Autodesk Inventor part; units mm, degrees
ref_plane "YZ Plane" through (0, 0, 0) normal (1, 0, 0) x (0, 1, 0)
ref_plane "XZ Plane" through (0, 0, 0) normal (0, 1, 0) x (-1, 0, 0)
ref_plane "XY Plane" through (0, 0, 0) normal (0, 0, 1) x (1, 0, 0)
sketch "Skizze2" plane through (0, 0, 0) normal (0, 1, 0) x (-1, 0, 0)
  line L0 (18.5, 0) -> (9.25, -16.0215)
  line L1 (9.25, -16.0215) -> (-9.25, -16.0215)
  line L2 (-9.25, -16.0215) -> (-18.5, 0)
  line L3 (-18.5, 0) -> (-9.25, 16.0215)
  line L4 (-9.25, 16.0215) -> (9.25, 16.0215)
  line L5 (9.25, 16.0215) -> (18.5, 0)
  point P0 (0, 0)
  point P1 (0, 0)
  dimension "d8" = 37
extrude "Extrusion1" add sketch "Skizze2" along normal blind 5
sketch "Skizze4" plane through (0, 0, 0) normal (0, 0, 1) x (1, 0, 0)
  line L0 (9.25, 5) -> (-9.25, 5)
  line L1 (-9.25, 5) -> (-18.5, 5)
  line L2 (18.5, 5) -> (9.25, 5)
  arc A0 (-18.5, 5) -> (-13.5631, 9.2083) centre (-18.5, 10) ccw
  line L3 (-13.5631, 9.2083) -> (-11.8486, 19.9)
  arc A1 (0, 30) -> (-11.8486, 19.9) centre (0, 18) ccw
  line L4 (0, 30) -> (0, 0)
  line L5 (9.25, 0) -> (-9.25, 0)
  point P0 (0, 5)
  dimension "d11" = 12
  dimension "d12" = 5
  dimension "d13" = 30
revolve "Umdrehung1" add sketch "Skizze4" angle 360 about axis through (0, 30, 0) along (0, -1, 0)
sketch "Skizze5" plane through (0, 0, 0) normal (0, -1, 0) x (1, 0, 0)
  line L0 (-9.25, 16.0215) -> (9.25, 16.0215)
  line L1 (-18.5, 0) -> (-9.25, 16.0215)
  line L2 (-9.25, -16.0215) -> (-18.5, 0)
  line L3 (9.25, -16.0215) -> (-9.25, -16.0215)
  line L4 (18.5, 0) -> (9.25, -16.0215)
  line L5 (9.25, 16.0215) -> (18.5, 0)
  arc A0 (-18.5, 0) -> (-9.25, -16.0215) centre (0, 0) ccw
  arc A1 (-9.25, 16.0215) -> (-18.5, 0) centre (0, 0) ccw
  arc A2 (9.25, 16.0215) -> (-9.25, 16.0215) centre (0, 0) ccw
  arc A3 (18.5, 0) -> (9.25, 16.0215) centre (0, 0) ccw
  arc A4 (9.25, -16.0215) -> (18.5, 0) centre (0, 0) ccw
  line L6 (9.25, -16.0215) -> (-9.25, -16.0215)
  arc A5 (-9.25, -16.0215) -> (9.25, -16.0215) centre (0, 0) ccw
  point P0 (0, 0)
extrude "Extrusion4" cut sketch "Skizze5" against normal up to surface contours A2 L0 | L1 A1 | A3 L5 | L2 A0 | A4 L4 | L3 A5
sketch "Skizze6" plane through (0, 0, 0) normal (0, -1, 0) x (1, 0, 0)
  point P0 (0, 0)
  point P1 (0, 0)
hole "Bohrung1" at (0, 0, 0) direction (0, 1, 0) diameter 8.376 depth 25 tip angle 118
properties part number "Spinner" material "Bronze, Cast"
Work out the finished part from the listing and answer in its coordinate system (mm). A direction names the side the tool comes from. Round coordinates to 2 decimals unless told otherwise and drop trailing zeros. Write each loop counter-clockwise with the first axis right and the second up, starting at its lowest first coordinate (ties: lowest second). Pieces come first, ordered by that corner, then holes.
1) A tool of negligible diameter and unlimited length cuts with its end or side. For faces 4 (the cylindrical face through (-2.83, 12.675, 3.087)), 5 (the flat face through (13.94, 2.79, 7.9)), from which of +Z, -Z, +X, -X, +Y, -Y can it reach the whole face along a straight path? Write none if from no direction.
2) A cutting plane is placed at A-A (y = 3). Give the vertices of the cut face in (x, z).
3) Straight lines are drawn through the part: line 1 (Z direction, x = 1, y = 23.5); line 2 (Z direction, x = 0, y = 8.75); line 3 (X direction, y = 15.5, z = 0). For each, find the intervals that lie inside material, in ascending order.
4) Given pin 1 Ø1 at (y, z) = (16, 4) entering from +X; pin 2 Ø3 at (x, y) = (-6.5, 25) entering from -Z; pin 3 Ø6 at (x, z) = (-12, -7) entering from +Y; pin 4 Ø3 at (x, y) = (14, 20) entering from -Z, each flat-ended and moving along its own axis, determine where each tip first touches the part or whether it passes through.
5) The mould has two halves that part along Z. Classify faces 1 (the conical face through (0.49, 27.08, 0.54)), 2 (the flat face through (0, 3, 16.022)), 3 (the flat face through (-13.94, 2.79, -7.9)): pulls with the +Z half, pulls with the -Z half, needs draft (parallel to the pull), parting line crosses it, or undercut.
6) A cutting plane is placed at B-B (y = 12). Give the vertices of the cut face in (x, z), plus the area to 3 significant figures.
Completed:
1. face 4: -Y
1. face 5: +Z, +X, +Y, -Y
2. outline: (-18.5, 0) - (-9.25, -16.02) - (9.25, -16.02) - (18.5, 0) - (9.25, 16.02) - (-9.25, 16.02) - close; hole circle Ø8.38 at (0, 0)
3. line 1: z = -10.62 to -4.07, 4.07 to 10.62
3. line 2: z = -13.66 to -4.19, 4.19 to 13.66
3. line 3: x = -12.55 to -4.19, 4.19 to 12.55
4. pin 1: stops at x = 11.99
4. pin 2: stops at z = -8.9
4. pin 3: stops at y = 23.04
4. pin 4: passes through
5. face 1: undercut
5. face 2: pulls with the +Z half
5. face 3: pulls with the -Z half
6. outline: circle Ø26.23 at (0, 0); hole circle Ø8.38 at (0, 0)
6. area: 485 mm2
